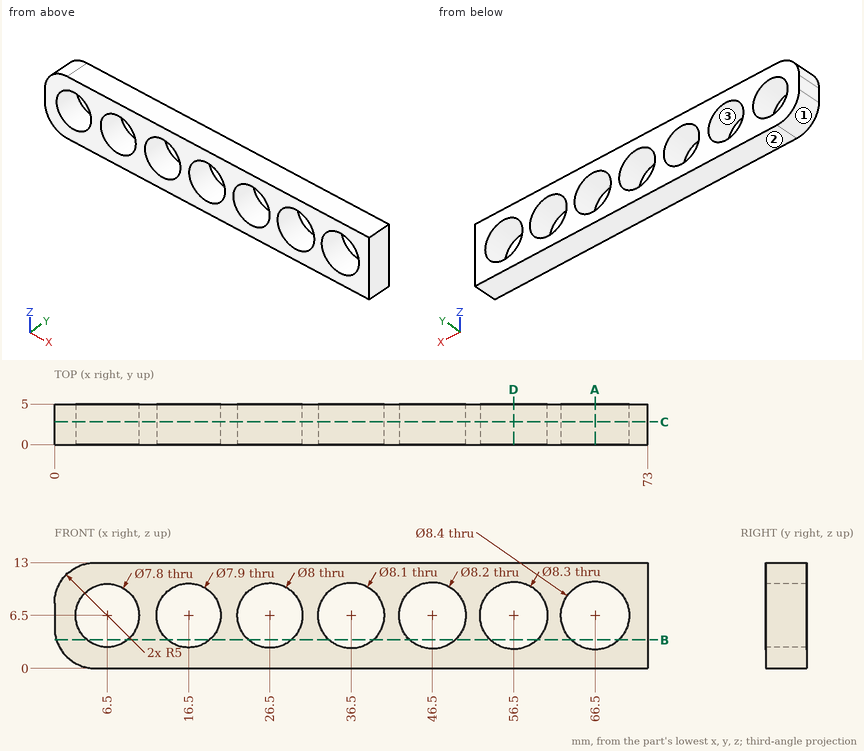
Source: three-view drawing plus pictorial views. Frame: mm from the lowest corner of the part. Give positions to 0.01 mm unless a question says otherwise; leave off trailing zeros. Loops run counter-clockwise (first coordinate to the right, second up) from the corner with the lowest first, then second, coordinate; pieces in that order, holes last. Notation, with made-up numbers: M 24.25,49.5 L 70.25,49.5 A15 cw 70.25,58.5 Z; hole C -19,71.5 d11. An arc over 180 degrees is marked long. Put each result on its own line as item: value.
Q1. Pin query (flat end, axial travel): P1, Ø6.5, axis at x = 26.5, z = 6.5, coming from the +Y side; P2, Ø3, axis at y = 3.5, z = 3, coming from the -X side. Return the tip coordinate at first contact, or that it passes through.
Response values:
P1: passes through
P2: stops at x = 0.03
Q2. Line query: probe 1 along Z at (x, y) = (36.5, 1.4); probe 2 along Z at (x, y) = (46.5, 3.5); probe 3 along X at (y, z) = (1.65, 12.25). Output: solid intervals per line, ascending. Write a range as [from, to].
Response values:
probe 1: z = [0, 2.45], [10.55, 13]
probe 2: z = [0, 2.4], [10.6, 13]
probe 3: x = [2.37, 73]
Q3. Section D-D (x = 56.5). Return the cut outline in (y, z).
Response values:
outline: M 0,0 L 5,0 L 5,2.35 L 0,2.35 Z; M 0,10.65 L 5,10.65 L 5,13 L 0,13 Z
Q4. Mould query, pull axis X, two halves, no side actions, for the marked faces 1, 2 and 3. Classes: released by +X, released by -X, zero draft, split by the parting line, or undercut.
Response values:
face 1: released by -X
face 2: zero draft
face 3: undercut
Q5. Section B-B (z = 3.5). Count the separate pieces of the cut face and the enclosed holes in it, and give its area (3 significant figures).
Response values:
separate pieces: 8
enclosed holes: 0
area: 174 mm²
Q6. Section C-C (y = 2.8). Return the cut outline in (x, z).
Response values:
outline: M 0,5 A5 ccw 5,0 L 73,0 L 73,13 L 5,13 A5 ccw 0,8 Z; hole C 6.5,6.5 d7.8; hole C 16.5,6.5 d7.9; hole C 26.5,6.5 d8; hole C 36.5,6.5 d8.1; hole C 46.5,6.5 d8.2; hole C 56.5,6.5 d8.3; hole C 66.5,6.5 d8.4
Q7. Section A-A (x = 66.5). Return the cut outline in (y, z).
Response values:
outline: M 0,0 L 5,0 L 5,2.3 L 0,2.3 Z; M 0,10.7 L 5,10.7 L 5,13 L 0,13 Z
